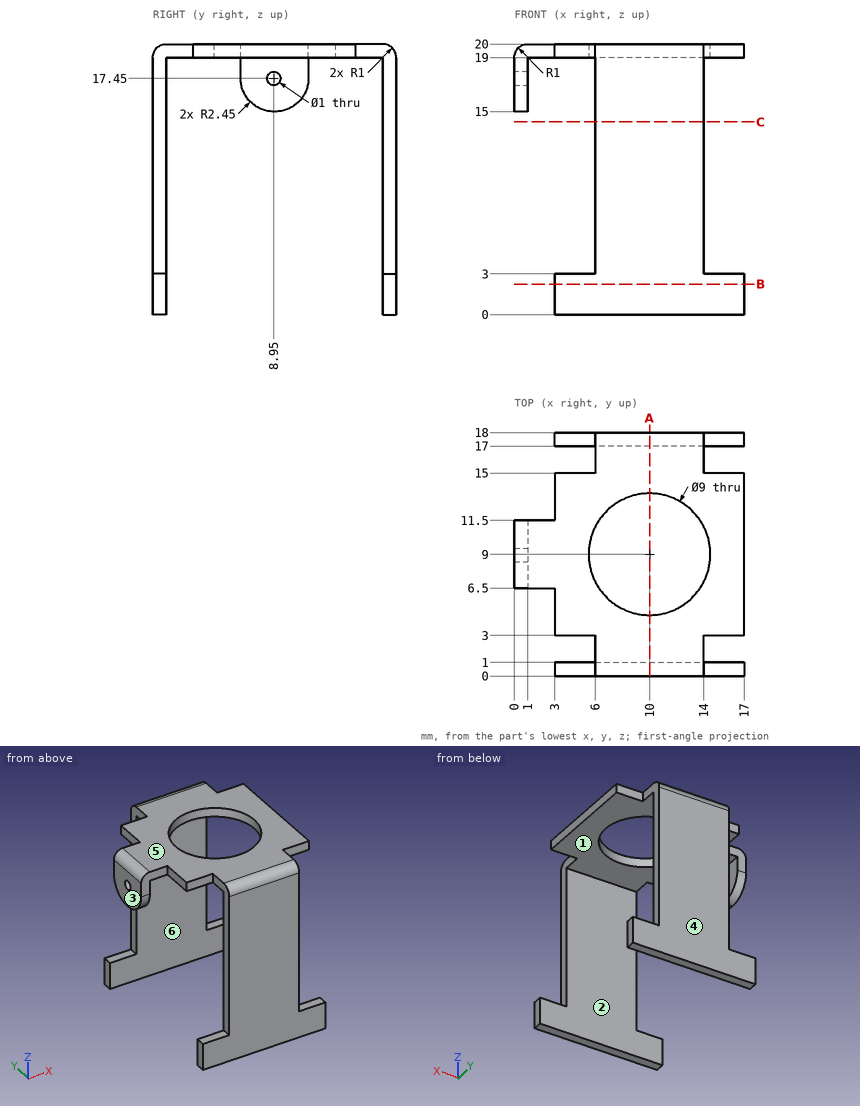
Job drawing, mm, ordinate dimensions from the low corner. One solid piece. A direction names the side the tool comes from. Round coordinates to 2 decimals unless told otherwise and drop trailing zeros. Order: outer loops, then holes, each group sorted by start corner. A loop starts at its lowest first (then second) coordinate and runs counter-clockwise, first axis right, second up. Notation, with made-up numbers: (77.5, 36) - (132.5, 36) arc R12 ccw to (132.5, 52) - close; hole circle Ø1 at (-19.75, -8). An arc over 180 degrees is marked (long way). Use CSV: the item, a comma, the result in double quotes. Start each with the question number.
1) Pin check, flat tips, straight feed: pin 1 Ø6 at (x, z) = (2.5, 14.5) entering from -Y; pin 2 Ø1.5 at (y, z) = (1.5, 13) entering from -X; pin 3 Ø0.8 at (x, z) = (4.5, 19.5) entering from +Y; pin 4 Ø5.5 at (x, y) = (10, 9) entering from -Z. Stop position of each tip, or through.
2) Tool access for the marked faces 1, 2 and 3: list every direction of +Z, -Z, +X, -X, +Y, -Y with a clear straight run to the whole face (end or side of a thin tool).
3) Saw through at B-B (z = 2.25). List the corners of the cut face in (x, y), and give its area (3 significant figures).
4) Two-plate mould, pull along Y, no slides. Class the marked faces 4, 5 and 6: pulls with the +Y half, pulls with the -Y half, needs draft (parallel to the pull), parting line crosses it, or undercut.
5) Saw through at A-A (x = 10). List the corners of the cut face in (y, z).
6) Saw through at C-C (z = 14.25). List the corners of the cut face in (x, y).
7) Wall check: L1, parallel to Y at x = 5.25, z = 2; L2, parallel to Y at x = 0.5, z = 17.45; L3, parallel to X at y = 17.25, z = 16.25. Give the ranges that are in metal, low to high. Write a range as [from, to].
Values follow:
1,pin 1,"stops at y = 6.53"
1,pin 2,"stops at x = 6"
1,pin 3,"stops at y = 15"
1,pin 4,"passes through"
2,face 1,"-Z, +X"
2,face 2,"-Z, +X, -X"
2,face 3,"+Z, -Z, -X, +Y, -Y"
3,outline,"(3, 0) - (17, 0) - (17, 1) - (3, 1) - close; (3, 17) - (17, 17) - (17, 18) - (3, 18) - close"
3,area,"28.0 mm2"
4,face 4,"pulls with the +Y half"
4,face 5,"needs draft"
4,face 6,"undercut"
5,outline,"(0, 0) - (1, 0) - (1, 19) - (4.5, 19) - (4.5, 20) - (1, 20) arc R1 ccw to (0, 19) - close; (13.5, 19) - (17, 19) - (17, 0) - (18, 0) - (18, 19) arc R1 ccw to (17, 20) - (13.5, 20) - close"
6,outline,"(6, 0) - (14, 0) - (14, 1) - (6, 1) - close; (6, 17) - (14, 17) - (14, 18) - (6, 18) - close"
7,L1,"y = [0, 1], [17, 18]"
7,L2,"y = [6.5, 8.45], [9.45, 11.5]"
7,L3,"x = [6, 14]"
